Check sheet for the modelled part. Datum: model origin and axes. Units: mm. Give positions to 0.01 mm unless a question says otherwise; leave off trailing zeros. Write each loop counter-clockwise with the first axis right and the second up, starting at its lowest first coordinate (ties: lowest second). Pieces come first, ordered by that corner, then holes. Notation, with made-up numbers: M 75.25,24.5 L 131.25,24.5 A21 ccw 131.25,47.5 Z; hole C 67.25,86.5 d11. An arc over 180 degrees is marked long. Write item = value, one per line. Start each with the question number.
1) Go/stop test with flat-tipped pins: pin 1 (6 mm diameter, centred on x = -69.5, y = 3, fed in from +Z); pin 2 (7.5 mm diameter, centred on x = -260, z = 0, fed in from +Y); pin 3 (4 mm diameter, centred on x = -135.5, y = -1, fed in from -Z); pin 4 (4 mm diameter, centred on y = 2, z = 6, fed in from +X). Record where each tip stops, or that it passes through.
2) Cross-section at A-A, the plane x = -260. Record the cut outline in (y, z) (3 decimals).
3) Scan lines: line 1 along Z through (x, y) = (-260, 1.5); line 2 along Y through (x, z) = (-94.5, 7.5); line 3 along Z through (x, y) = (0, 4.7). Record each from-to range of solid material in increasing order. Write a range as [from, to].
```python
from build123d import *

# Parameters (mm, degrees)
CROQUIS1_R                                           = 4.05
SALIENTE_EXTRUIR1_DEPTH                              = 5
CROQUIS2_R                                           = 10
SALIENTE_EXTRUIR2_DEPTH                              = 10
REDONDEO8_R                                          = 10
REFRENTADO_PARA_TORNILLO_CON_CABEZA_PLAN_D           = 8.1
REFRENTADO_PARA_TORNILLO_CON_CABEZA_PLAN_CBORE_D     = 12.4
REFRENTADO_PARA_TORNILLO_CON_CABEZA_PLAN_CBORE_DEPTH = 1.2
REDONDEO9_R                                          = 4
REFRENTADO_PARA_TORNILLO_CON_CABEZA_2_D              = 8.1
REFRENTADO_PARA_TORNILLO_CON_CABEZA_2_CBORE_D        = 12.4
REFRENTADO_PARA_TORNILLO_CON_CABEZA_2_CBORE_DEPTH    = 1.2


with BuildPart() as part:
    # Croquis1 → Saliente-Extruir1 (new, symmetric)
    with BuildSketch(Plane(origin=(0, 0, 0), x_dir=(-1, 0, 0), z_dir=(0, 1, 0))):
        with BuildLine():
            Line((52.388821078, 22.035902101), (260.523173553, 7.481730377))
            ThreePointArc((260.523173553, 7.481730377), (267.481730377, -0.523173553), (259.476826447, -7.481730377))
            Line((259.476826447, -7.481730377), (51.342473972, 7.072441348))
            ThreePointArc((51.342473972, 7.072441348), (26.697288319, 4.552818898), (4.339230902, -6.117276778))
            ThreePointArc((4.339230902, -6.117276778), (-6.117276778, -4.339230902), (-4.339230902, 6.117276778))
            ThreePointArc((-4.339230902, 6.117276778), (22.644631497, 18.994978455), (52.388821078, 22.035902101))
        make_face()
        with Locations(Location((0, 0, 0), (0, 0, 90))):
            Circle(CROQUIS1_R, mode=Mode.SUBTRACT)
        with Locations(Location((260, 0, 0), (0, 0, 90))):
            Circle(CROQUIS1_R, mode=Mode.SUBTRACT)
    extrude(amount=SALIENTE_EXTRUIR1_DEPTH, both=True)

    # Croquis2 → Saliente-Extruir2 (add)
    with BuildSketch(Plane(origin=(0, 5, 0), x_dir=(-1, 0, 0), z_dir=(0, 1, 0))):
        Circle(CROQUIS2_R)
        with Locations((260, 0)):
            Circle(CROQUIS2_R)
    extrude(amount=-SALIENTE_EXTRUIR2_DEPTH)

    # Redondeo8
    redondeo8_edges = [part.edges().sort_by_distance(p)[0] for p in [
        (-1.45671448, 0, 9.893330224),
        (-253.924907568, 0, 7.943126082),
        (-9.62840856, 0, -2.700694098),
        (-252.878560462, 0, -7.020334672),
    ]]
    fillet(redondeo8_edges, radius=REDONDEO8_R)

    # Refrentado para tornillo con cabeza plan (through all)
    with Locations(Plane(origin=(0, 5, 0), x_dir=(-1, 0, 0), z_dir=(0, 1, 0))):
        with Locations((0, 0)):
            CounterBoreHole(REFRENTADO_PARA_TORNILLO_CON_CABEZA_PLAN_D / 2, REFRENTADO_PARA_TORNILLO_CON_CABEZA_PLAN_CBORE_D / 2, REFRENTADO_PARA_TORNILLO_CON_CABEZA_PLAN_CBORE_DEPTH)

    # Redondeo9
    redondeo9_edges = [part.edges().sort_by_distance(p)[0] for p in [
        (-150.580214018, 5, 0.133062562),
        (-27.298211365, 5, 20.16419235),
        (-31.522388758, 5, 5.730111954),
        (-31.522388758, -5, 5.730111954),
        (8.493504141, 5, -5.278293987),
        (8.493504141, -5, -5.278293987),
        (-269.975640503, -5, -0.697564737),
        (-269.975640503, 5, -0.697564737),
        (-151.626561124, 5, 15.096523316),
        (-151.626561124, -5, 15.096523316),
        (-27.298211365, -5, 20.16419235),
        (-10.473813488, -5, -2.625536281),
        (-10.473813488, 5, -2.625536281),
        (-252.289713604, 5, -7.297475528),
        (-252.289713604, -5, -7.297475528),
        (-253.38036188, -5, 8.299521464),
        (-253.38036188, 5, 8.299521464),
        (-1.68943962, 5, 10.362079146),
        (-1.68943962, -5, 10.362079146),
        (-150.580214018, -5, 0.133062562),
    ]]
    fillet(redondeo9_edges, radius=REDONDEO9_R)

    # Refrentado para tornillo con cabeza  2 (through all)
    with Locations(Plane.XZ.offset(5)):
        with Locations((-260, 0)):
            CounterBoreHole(REFRENTADO_PARA_TORNILLO_CON_CABEZA_2_D / 2, REFRENTADO_PARA_TORNILLO_CON_CABEZA_2_CBORE_D / 2, REFRENTADO_PARA_TORNILLO_CON_CABEZA_2_CBORE_DEPTH)


solid = part.part
```
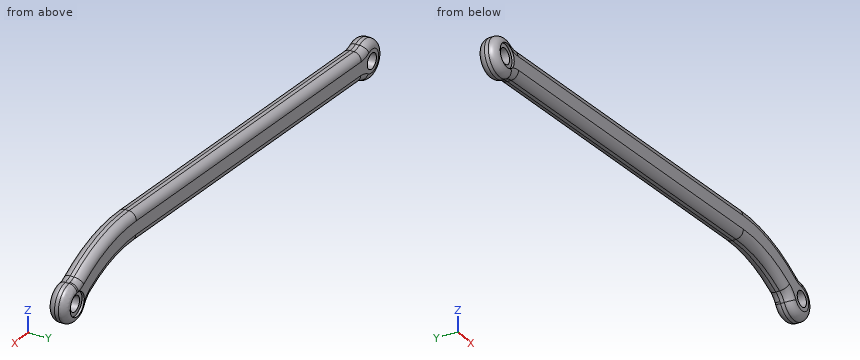
Reply:
q1.pin_1 = 21
q1.pin_2 = through
q1.pin_3 = 1.05
q1.pin_4 = 9.1
q2.outline = M -4.995,-6.2 A4 ccw -1,-10 L 1,-10 A4 ccw 5,-6 L 5,-4.05 L -3.8,-4.05 L -3.8,-6.2 Z; M -4.995,6.2 L -3.8,6.2 L -3.8,4.05 L 5,4.05 L 5,6 A4 ccw 1,10 L -1,10 A4 ccw Z
q3.line_1 = [-9.97, -4.05], [4.05, 9.97]
q3.line_2 = [-4.96, 4.96]
q3.line_3 = [-7.53, -6.2], [6.2, 7.55]
